```python
from build123d import *

# Parameters (mm, degrees)
EXTRUDE_1_DEPTH     = 25
SKETCH_3_R          = 7.5
CUT_EXTRUDE_1_DEPTH = 5
SKETCH_5_R          = 7.5
CUT_EXTRUDE_2_DEPTH = 5
FILLET_1_R          = 0.5


with BuildPart() as part:
    # 草图1 → 凸台-拉伸1 (new body, symmetric)
    with BuildSketch(Plane.XY):
        with BuildLine():
            Line((0, 10), (0, 90))
            ThreePointArc((0, 90), (-2.928932188, 97.071067812), (-10, 100))
            Line((-10, 100), (-87, 100))
            ThreePointArc((-87, 100), (-89.5, 97.5), (-87, 95))
            Line((-87, 95), (-10, 95))
            ThreePointArc((-10, 95), (-6.464466094, 93.535533906), (-5, 90))
            Line((-5, 90), (-5, 10))
            ThreePointArc((-5, 10), (-6.464466094, 6.464466094), (-10, 5))
            Line((-10, 5), (-47.320508076, 5))
            ThreePointArc((-47.320508076, 5), (-48.614603301, 5.170370869), (-49.820508076, 5.669872981))
            Line((-49.820508076, 5.669872981), (-92.5, 30.310889132))
            ThreePointArc((-92.5, 30.310889132), (-95.915063509, 29.395825623), (-95, 25.980762114))
            Line((-95, 25.980762114), (-52.320508076, 1.339745962))
            ThreePointArc((-52.320508076, 1.339745962), (-49.908698527, 0.340741737), (-47.320508076, 0))
            Line((-47.320508076, 0), (-10, 0))
            ThreePointArc((-10, 0), (-2.928932188, 2.928932188), (0, 10))
        make_face()
    extrude(amount=EXTRUDE_1_DEPTH, both=True)

    # 草图3 → 切除-拉伸1 (cut)
    with BuildSketch(Plane(origin=(-10, -17.320508076, 0), x_dir=(0.866025404, -0.5, 0), z_dir=(0.5, 0.866025404, 0))):
        with Locations((-75.358983849, 0)):
            Circle(SKETCH_3_R)
    extrude(amount=-CUT_EXTRUDE_1_DEPTH, mode=Mode.SUBTRACT)

    # 草图5 → 切除-拉伸2 (cut)
    with BuildSketch(Plane(origin=(0, 100, 0), x_dir=(1, 0, 0), z_dir=(0, 1, 0))):
        with Locations((-55.262794416, 0)):
            Circle(SKETCH_5_R)
    extrude(amount=-CUT_EXTRUDE_2_DEPTH, mode=Mode.SUBTRACT)

    # 圆角1
    fillet_1_edges = [part.edges().sort_by_distance(p)[0] for p in [
        (-89.5, 97.5, 25),
        (0, 50, -25),
        (-2.928932188, 2.928932188, -25),
        (-28.660254038, 0, -25),
        (-48.5, 95, 25),
        (-49.908698527, 0.340741737, -25),
        (-73.660254038, 13.660254038, -25),
        (-95.915063509, 29.395825623, -25),
        (-71.160254038, 17.990381057, -25),
        (-48.614603301, 5.170370869, -25),
        (-28.660254038, 5, -25),
        (-6.464466094, 6.464466094, -25),
        (-5, 50, -25),
        (-6.464466094, 93.535533906, -25),
        (-48.5, 95, -25),
        (-6.464466094, 93.535533906, 25),
        (-89.5, 97.5, -25),
        (-48.5, 100, -25),
        (-2.928932188, 97.071067812, -25),
        (-5, 50, 25),
        (-6.464466094, 6.464466094, 25),
        (-28.660254038, 5, 25),
        (-48.614603301, 5.170370869, 25),
        (-71.160254038, 17.990381057, 25),
        (-95.915063509, 29.395825623, 25),
        (-73.660254038, 13.660254038, 25),
        (-2.928932188, 97.071067812, 25),
        (-49.908698527, 0.340741737, 25),
        (-28.660254038, 0, 25),
        (-2.928932188, 2.928932188, 25),
        (0, 50, 25),
        (-48.5, 100, 25),
    ]]
    fillet(fillet_1_edges, radius=FILLET_1_R)


solid = part.part
```
Geometry: final body of the model. Coordinates: model frame, mm. A direction names the side the tool comes from. Coordinates: 2 decimals unless noted, no trailing zeros. Order: outer loops, then holes, each group sorted by start corner. A loop starts at its lowest first (then second) coordinate and runs counter-clockwise, first axis right, second up. Notation, with made-up numbers: M 21,59.5 L 68,59.5 A32 cw 68,87.5 Z; hole C 28,-19.75 d10. An arc over 180 degrees is marked long. Answer in a Markdown table with one row per item. Add a question column.
Q1. Line query: L1, parallel to Y at x = -40.5, z = -23; L2, parallel to X at y = 63, z = 0; L3, parallel to Y at x = -71, z = 16. Output: solid intervals per line, ascending.
Q2. Section query C-C on z = 19. Return the cut outline in (x, y), and give its area (3 significant figures).
Q3. Section query B-B on y = 71. Return the cut outline in (x, z).
Q4. Section query A-A on x = -24. Return the cut outline in (y, z).
Q5. Reachability of faces 5 (the cylindrical face through (-7, 94, 0)), 6 (the cylindrical face through (-73.29, 13.61, -24.85)), 7 (the flat face through (-69.217, 11.095, 0.343)), 8 (the flat face through (-28, 5, 0)), 9 (the cylindrical face through (-71.53, 18.03, 24.86)) from +Z, -Z, +X, -X, +Y, -Y: full face, straight path, thin tool, end or side. Return the list, or none.
Q6. Contact query for flat-ended pins moving along their axis: P1, Ø2, axis at y = 37, z = 15.5, coming from the -X side; P2, Ø6, axis at y = 20.5, z = 8, coming from the -X side. Output: stop coordinate, or through.
Q7. Mould query, pull axis Y, two halves, no side actions, for faces 1 (the cylindrical face through (-62.756, 97.535, -0.33)), 2 (the cylindrical face through (-3.01, 2.85, 0.34)), 3 (the cylindrical face through (-95.89, 29.44, 0.34)), 4 (the cylindrical face through (-71.53, 18.04, -24.85)). Classes: released by +Y, released by -Y, zero draft, split by the parting line, or undercut.
Completed:
| question | item | result |
|---|---|---|
| 1 | L1 | y = 0 to 5, 95 to 100 |
| 1 | L2 | x = -5 to 0 |
| 1 | L3 | y = 12.12 to 17.9, 95 to 100 |
| 2 | outline | M -95,25.98 L -52.32,1.34 A10 ccw -47.32,0 L -10,0 A10 ccw 0,10 L 0,90 A10 ccw -10,100 L -87,100 A2.5 ccw -87,95 L -10,95 A5 cw -5,90 L -5,10 A5 cw -10,5 L -47.32,5 A5 cw -49.82,5.67 L -92.5,30.31 A2.5 ccw Z |
| 2 | area | 1,380 mm2 |
| 3 | outline | M -5,-24.5 A0.5 ccw -4.5,-25 L -0.5,-25 A0.5 ccw 0,-24.5 L 0,24.5 A0.5 ccw -0.5,25 L -4.5,25 A0.5 ccw -5,24.5 Z |
| 4 | outline | M 0,-24.5 A0.5 ccw 0.5,-25 L 4.5,-25 A0.5 ccw 5,-24.5 L 5,24.5 A0.5 ccw 4.5,25 L 0.5,25 A0.5 ccw 0,24.5 Z; M 95,-24.5 A0.5 ccw 95.5,-25 L 99.5,-25 A0.5 ccw 100,-24.5 L 100,24.5 A0.5 ccw 99.5,25 L 95.5,25 A0.5 ccw 95,24.5 Z |
| 5 | face 5 | +Z, -Z, -X |
| 5 | face 6 | -Z, -X, -Y |
| 5 | face 7 | +Z, -Z, -X, -Y |
| 5 | face 8 | +Z, -Z |
| 5 | face 9 | +Z |
| 6 | P1 | stops at x = -5 |
| 6 | P2 | stops at x = -90.7 |
| 7 | face 1 | zero draft |
| 7 | face 2 | released by -Y |
| 7 | face 3 | split by the parting line |
| 7 | face 4 | undercut |
